For this review, take the finished solid that the model builds, in its own axes (mm). A direction names the side the tool comes from. Give positions to 0.01 mm unless a question says otherwise; leave off trailing zeros. Order: outer loops, then holes, each group sorted by start corner. A loop starts at its lowest first (then second) coordinate and runs counter-clockwise, first axis right, second up. Notation, with made-up numbers: M 34.5,-13.5 L 85.5,-13.5 A25 ccw 85.5,4.5 Z; hole C 53.5,87 d9. An arc over 180 degrees is marked long. Use CSV: the item, a comma, the result in double quotes. Start each with the question number.
(1) Clearance check with a flat-ended pin moving along its axis: P1, Ø2, axis at x = 171.5, z = -11.5, coming from the +Y side. State where the tip first meets the part, or that it passes through.
(2) Tool access review of faces 1 (the face through (104, 117, -12.033)), 2 (the face through (86.458, 211.606, -9.229)): name each direction out of +Z, -Z, +X, -X, +Y, -Y from which nothing blocks a thin tool from reaching the whole face with its end or side.
(3) Draft analysis for pull direction X (two halves, no side actions). For faces 3 (the face through (28.41, 225.96, -9.31)), 4 (the face through (140.15, 213.83, -9.23)), 5 (the face through (106, 0, -9)), state which applies: pulls with the +X half, pulls with the -X half, needs draft (parallel to the pull), parting line crosses it, or undercut.
(4) Consider section C-C (x = 168). Write out the cut boundary in (y, z).
(5) Consider section A-A (x = 45). Write out the cut boundary in (y, z).
(6) Consider section B-B (z = -8.15). Write out the cut boundary in (x, y) (1 decimal).
(7) Wall thickness on L1, parallel to Y at x = 76, z = -7.5; L2, parallel to Y at x = 112, z = -7.5; L3, parallel to X at y = 189, z = -8.3: over which ranges is each line inside the solid? List them lowest first. Write a range as from..to.
Solid Edge part; units mm, degrees
sketch "Sketch1" plane through (0, 0, 0) normal (0, -1, 0) x (1, 0, 0)
  line L0 (17, -12.0333) -> (193, -12.0333)
  line L1 (193, -12.0333) -> (193, -6.5021)
  line L2 (193, -6.5021) -> (17, -6.5021)
  line L3 (17, -6.5021) -> (17, -12.0333)
extrude "Protrusion1" add sketch "Sketch1" against normal blind 237.9836
fillet "Round_1" radius 40 1 edges at (17, 237.9836, -9.2677)
fillet "Round_1" radius 30 1 edges at (193, 237.9836, -9.2677)
sketch "Sketch2" plane through (105, 118.9918, -6.5021) normal (0, 0, 1) x (1, 0, 0)
  arc A0 (28.6296, 93.6158) -> (41.4349, 93.3666) centre (34.7502, 78.9918) cw
  arc A1 (41.4349, 93.3666) -> (49.8683, 93.3666) centre (45.6516, 102.4341) ccw
  arc A2 (49.8683, 64.617) -> (41.4349, 64.617) centre (45.6516, 55.5495) ccw
  arc A3 (28.6296, 64.3678) -> (20.9081, 64.3678) centre (24.7689, 55.1432) ccw
  arc A4 (7.808, 64.7578) -> (-0.9972, 64.7578) centre (3.4054, 55.7791) ccw
  arc A5 (-14.4194, 64.5069) -> (-22.5474, 64.5069) centre (-18.4834, 55.3699) ccw
  arc A6 (-22.5474, 64.5069) -> (-34.8185, 64.249) centre (-28.99, 78.9918) cw
  arc A7 (-34.8185, 64.249) -> (-42.1715, 64.249) centre (-38.495, 54.9494) ccw
  arc A8 (-42.1715, 93.7346) -> (-34.8185, 93.7346) centre (-38.495, 103.0343) ccw
  arc A9 (-22.5474, 93.4768) -> (-14.4194, 93.4768) centre (-18.4834, 102.6137) ccw
  arc A10 (-14.4194, 93.4768) -> (-0.9972, 93.2259) centre (-7.9768, 78.9918) cw
  arc A11 (-0.9972, 93.2259) -> (7.808, 93.2259) centre (3.4054, 102.2045) ccw
  arc A12 (7.808, 93.2259) -> (20.9081, 93.6158) centre (14.7876, 78.9918) cw
  arc A13 (20.9081, 93.6158) -> (28.6296, 93.6158) centre (24.7689, 102.8405) ccw
  arc A14 (49.8683, 93.3666) -> (49.8683, 64.617) centre (56.5531, 78.9918) cw
  arc A15 (41.4349, 64.617) -> (28.6296, 64.3679) centre (34.7502, 78.9918) cw
  arc A16 (20.9081, 64.3678) -> (7.808, 64.7578) centre (14.7876, 78.9918) cw
  arc A17 (-0.9972, 64.7578) -> (-14.4194, 64.5068) centre (-7.9768, 78.9918) cw
  arc A18 (-42.1715, 64.249) -> (-42.1715, 93.7346) centre (-48, 78.9918) cw
  arc A19 (-34.8185, 93.7346) -> (-22.5474, 93.4767) centre (-28.99, 78.9918) cw
extrude "Cutout1" cut sketch "Sketch2" against normal up to vertex (79.4979 mm away)
Check result:
1,P1,"stops at y = 237.03"
2,face 1,"-Z, +X, -X, +Y, -Y"
2,face 2,"+Z, -Z"
3,face 3,"pulls with the -X half"
3,face 4,"undercut"
3,face 5,"needs draft"
4,outline,"M 0,-12.03 L 183.5,-12.03 L 183.5,-6.5 L 0,-6.5 Z; M 212.47,-12.03 L 237.56,-12.03 L 237.56,-6.5 L 212.47,-6.5 Z"
5,outline,"M 0,-12.03 L 187.62,-12.03 L 187.62,-6.5 L 0,-6.5 Z; M 208.34,-12.03 L 236.14,-12.03 L 236.14,-6.5 L 208.34,-6.5 Z"
6,outline,"M 17,0 L 193,0 L 193,208 A30 ccw 163,238 L 57,238 A40 ccw 17,198 Z; hole M 62.8,183.2 A10 cw 70.2,183.2 A15.9 ccw 82.5,183.5 A10 cw 90.6,183.5 A15.9 ccw 104,183.7 A10 cw 112.8,183.7 A15.9 ccw 125.9,183.4 A10 cw 133.6,183.4 A15.9 ccw 146.4,183.6 A10 cw 154.9,183.6 A15.9 ccw long 154.9,212.4 A10 cw 146.4,212.4 A15.9 ccw 133.6,212.6 A10 cw 125.9,212.6 A15.9 ccw 112.8,212.2 A10 cw 104,212.2 A15.9 ccw 90.6,212.5 A10 cw 82.5,212.5 A15.9 ccw 70.2,212.7 A10 cw 62.8,212.7 A15.9 ccw long Z"
7,L1,"y = 0..182.13, 213.84..237.98"
7,L2,"y = 0..184.1, 211.86..237.98"
7,L3,"x = 17..43.94, 174.62..193"
